from build123d import *

# Parameters (mm, degrees)
F0_R     = 20
F1_DEPTH = 9.4
F2_SIZE  = 1
F3_R     = 2.5


with BuildPart() as f1:
    # F0 (on Top) → F1 (new body)
    with BuildSketch(Plane.XY):
        Circle(F0_R)
    extrude(amount=F1_DEPTH)

    # F2
    f2_edges = [f1.edges().sort_by_distance(p)[0] for p in [
        (-20, 0, 9.4),
        (-20, 0, 0),
    ]]
    chamfer(f2_edges, length=F2_SIZE)

    # F3
    f3_edges = [f1.edges().sort_by_distance(p)[0] for p in [
        (-20, 0, 8.4),
        (-20, 0, 1),
    ]]
    fillet(f3_edges, radius=F3_R)


solid = f1.part
Read the model definition and answer for the solid it produces. Units are mm, in the model's axes. Coordinates: 2 decimals unless noted, no trailing zeros. Order: outer loops, then holes, each group sorted by start corner. A loop starts at its lowest first (then second) coordinate and runs counter-clockwise, first axis right, second up. Notation, with made-up numbers: M 44.25,-21.75 L 102.25,-21.75 A33 cw 102.25,16.25 Z; hole C -9.5,-3.75 d7. An arc over 180 degrees is marked long. Put each result on its own line as item: value. Start each with the question number.
Item 1: Consider probe 1 along X at (y, z) = (12.5, 5); probe 2 along Y at (x, z) = (-1, 2.75); probe 3 along Y at (x, z) = (4.5, 1.25). Determine where each line is inside the solid, lowest interval first. Write a range as [from, to].
Item 2: Section A-A, the plane z = 4.75 is taken. Determine the outline of the cut face in (x, y).
Item 3: Given pin 1 Ø5 at (x, z) = (11, 2) entering from -Y; pin 2 Ø4 at (x, z) = (10, 6) entering from -Y; pin 3 Ø5 at (y, z) = (-10.5, 2) entering from -X, each flat-ended and moving along its own axis, determine where each tip first touches the part or whether it passes through.
Computed:
1. probe 1: x = [-15.61, 15.61]
1. probe 2: y = [-19.97, 19.97]
1. probe 3: y = [-19.36, 19.36]
2. outline: C 0,0 d40
3. pin 1: stops at y = -18.1
3. pin 2: stops at y = -18.33
3. pin 3: stops at x = -18.33
